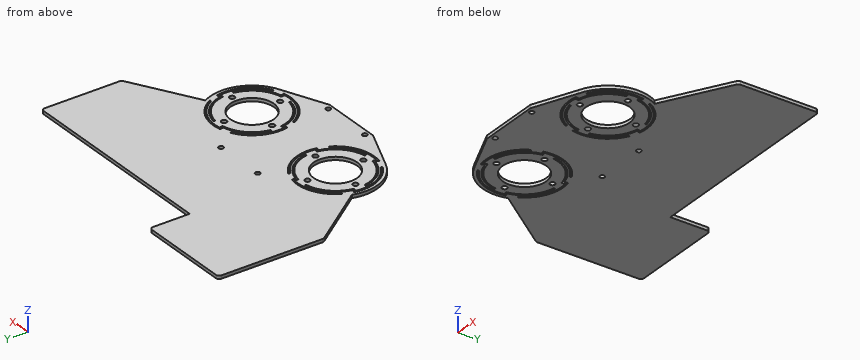
```python
from build123d import *

# Parameters (mm, degrees)
SKETCH_1_R          = 21
SKETCH_1_R_2        = 13.6
SKETCH_1_R_3        = 1.65
EXTRUDE_1_DEPTH     = 2
EXTRUDE_1_2_DEPTH   = 2
SKETCH_2_R          = 26.25
EXTRUDE_3_DEPTH     = 2
EXTRUDE_4_DEPTH     = 2
FILLET_1_R          = 2
SKETCH_4_R          = 1.5
CUT_EXTRUDE_1_DEPTH = 2


with BuildPart() as part:
    # Sketch 1 → Extrude 1 (new body)
    with BuildSketch(Plane.XY):
        with Locations((36.5, 0)):
            Circle(SKETCH_1_R)
        with Locations((36.5, 0)):
            Circle(SKETCH_1_R_2, mode=Mode.SUBTRACT)
        with Locations((19, 0)):
            Circle(SKETCH_1_R_3, mode=Mode.SUBTRACT)
        with Locations((36.5, 17.5)):
            Circle(SKETCH_1_R_3, mode=Mode.SUBTRACT)
        with Locations((54, 0)):
            Circle(SKETCH_1_R_3, mode=Mode.SUBTRACT)
        with Locations((36.5, -17.5)):
            Circle(SKETCH_1_R_3, mode=Mode.SUBTRACT)
    extrude(amount=EXTRUDE_1_DEPTH)

    # Sketch 2 → Extrude 3 (add)
    # profile 1 of 4: a face of its own
    with BuildSketch(Plane.XY):
        with Locations((36.5, 0)):
            Circle(SKETCH_2_R)
        with BuildLine():
            Line((58.229143493, 3.441558231), (57.241455152, 3.285123766))
            ThreePointArc((57.241455152, 3.285123766), (57.435264008, 1.64764101), (57.5, 0))
            ThreePointArc((57.5, 0), (57.435264008, -1.64764101), (57.241455152, -3.285123766))
            Line((57.241455152, -3.285123766), (58.229143493, -3.441558231))
            ThreePointArc((58.229143493, -3.441558231), (52.524161337, -15.074025787), (41.261671507, -21.478512157))
            Line((41.261671507, -21.478512157), (41.748660638, -23.675178173))
            ThreePointArc((41.748660638, -23.675178173), (26.251507153, -21.977963836), (14.989987295, -11.197403871))
            Line((14.989987295, -11.197403871), (15.876998129, -10.735655258))
            ThreePointArc((15.876998129, -10.735655258), (26.035211246, -20.761760434), (40.137101312, -22.963753919))
            Line((40.137101312, -22.963753919), (39.785123766, -20.741455152))
            ThreePointArc((39.785123766, -20.741455152), (36.5, -21), (33.214876234, -20.741455152))
            Line((33.214876234, -20.741455152), (33.058441769, -21.729143493))
            ThreePointArc((33.058441769, -21.729143493), (21.425974213, -16.024161337), (15.021487843, -4.761671507))
            Line((15.021487843, -4.761671507), (12.824821827, -5.248660638))
            ThreePointArc((12.824821827, -5.248660638), (14.522036164, 10.248492847), (25.302596129, 21.510012705))
            Line((25.302596129, 21.510012705), (25.764344742, 20.623001871))
            ThreePointArc((25.764344742, 20.623001871), (15.738239566, 10.464788754), (13.536246081, -3.637101312))
            Line((13.536246081, -3.637101312), (14.770856507, -3.441558231))
            Line((14.770856507, -3.441558231), (15.758544848, -3.285123766))
            ThreePointArc((15.758544848, -3.285123766), (15.5, 0), (15.758544848, 3.285123766))
            Line((15.758544848, 3.285123766), (14.770856507, 3.441558231))
            ThreePointArc((14.770856507, 3.441558231), (20.475838663, 15.074025787), (31.738328493, 21.478512157))
            Line((31.738328493, 21.478512157), (31.251339362, 23.675178173))
            ThreePointArc((31.251339362, 23.675178173), (46.748492847, 21.977963836), (58.010012705, 11.197403871))
            ThreePointArc((58.010012705, 11.197403871), (59.287546054, 8.293988476), (60.175178173, 5.248660638))
            ThreePointArc((60.175178173, 5.248660638), (58.477963836, -10.248492847), (47.697403871, -21.510012705))
            Line((47.697403871, -21.510012705), (47.235655258, -20.623001871))
            ThreePointArc((47.235655258, -20.623001871), (57.261760434, -10.464788754), (59.463753919, 3.637101312))
            Line((59.463753919, 3.637101312), (58.229143493, 3.441558231))
        make_face(mode=Mode.SUBTRACT)
    # profile 2 of 4: a face of its own
    with BuildSketch(Plane.XY):
        with BuildLine():
            Line((39.785123766, 20.741455152), (39.941558231, 21.729143493))
            ThreePointArc((39.941558231, 21.729143493), (51.574025787, 16.024161337), (57.978512157, 4.761671507))
            Line((57.978512157, 4.761671507), (60.175178173, 5.248660638))
            ThreePointArc((60.175178173, 5.248660638), (59.287546054, 8.293988476), (58.010012705, 11.197403871))
            Line((58.010012705, 11.197403871), (57.123001871, 10.735655258))
            ThreePointArc((57.123001871, 10.735655258), (46.964788754, 20.761760434), (32.862898688, 22.963753919))
            Line((32.862898688, 22.963753919), (33.214876234, 20.741455152))
            ThreePointArc((33.214876234, 20.741455152), (36.5, 21), (39.785123766, 20.741455152))
        make_face()
    # profile 3 of 4: a face of its own
    with BuildSketch(Plane.XY):
        with Locations((-36.5, 0)):
            Circle(SKETCH_2_R)
        with BuildLine():
            ThreePointArc((-31.738328493, 21.478512157), (-20.475838663, 15.074025787), (-14.770856507, 3.441558231))
            Line((-14.770856507, 3.441558231), (-15.758544848, 3.285123766))
            ThreePointArc((-15.758544848, 3.285123766), (-15.564735992, 1.64764101), (-15.5, 0))
            ThreePointArc((-15.5, 0), (-15.564735992, -1.64764101), (-15.758544848, -3.285123766))
            Line((-15.758544848, -3.285123766), (-14.770856507, -3.441558231))
            Line((-14.770856507, -3.441558231), (-13.536246081, -3.637101312))
            ThreePointArc((-13.536246081, -3.637101312), (-15.738239566, 10.464788754), (-25.764344742, 20.623001871))
            Line((-25.764344742, 20.623001871), (-25.302596129, 21.510012705))
            ThreePointArc((-25.302596129, 21.510012705), (-14.522036164, 10.248492847), (-12.824821827, -5.248660638))
            Line((-12.824821827, -5.248660638), (-15.021487843, -4.761671507))
            ThreePointArc((-15.021487843, -4.761671507), (-21.425974213, -16.024161337), (-33.058441769, -21.729143493))
            Line((-33.058441769, -21.729143493), (-33.214876234, -20.741455152))
            ThreePointArc((-33.214876234, -20.741455152), (-36.5, -21), (-39.785123766, -20.741455152))
            Line((-39.785123766, -20.741455152), (-40.137101312, -22.963753919))
            ThreePointArc((-40.137101312, -22.963753919), (-26.035211246, -20.761760434), (-15.876998129, -10.735655258))
            Line((-15.876998129, -10.735655258), (-14.989987295, -11.197403871))
            ThreePointArc((-14.989987295, -11.197403871), (-26.251507153, -21.977963836), (-41.748660638, -23.675178173))
            Line((-41.748660638, -23.675178173), (-41.261671507, -21.478512157))
            ThreePointArc((-41.261671507, -21.478512157), (-52.524161337, -15.074025787), (-58.229143493, -3.441558231))
            Line((-58.229143493, -3.441558231), (-57.241455152, -3.285123766))
            ThreePointArc((-57.241455152, -3.285123766), (-57.5, 0), (-57.241455152, 3.285123766))
            Line((-57.241455152, 3.285123766), (-58.229143493, 3.441558231))
            Line((-58.229143493, 3.441558231), (-59.463753919, 3.637101312))
            ThreePointArc((-59.463753919, 3.637101312), (-57.261760434, -10.464788754), (-47.235655258, -20.623001871))
            Line((-47.235655258, -20.623001871), (-47.697403871, -21.510012705))
            ThreePointArc((-47.697403871, -21.510012705), (-58.477963836, -10.248492847), (-60.175178173, 5.248660638))
            ThreePointArc((-60.175178173, 5.248660638), (-59.287546054, 8.293988476), (-58.010012705, 11.197403871))
            ThreePointArc((-58.010012705, 11.197403871), (-46.748492847, 21.977963836), (-31.251339362, 23.675178173))
            Line((-31.251339362, 23.675178173), (-31.738328493, 21.478512157))
        make_face(mode=Mode.SUBTRACT)
    # profile 4 of 4: a face of its own
    with BuildSketch(Plane.XY):
        with BuildLine():
            ThreePointArc((-39.785123766, 20.741455152), (-36.5, 21), (-33.214876234, 20.741455152))
            Line((-33.214876234, 20.741455152), (-32.862898688, 22.963753919))
            ThreePointArc((-32.862898688, 22.963753919), (-46.964788754, 20.761760434), (-57.123001871, 10.735655258))
            Line((-57.123001871, 10.735655258), (-58.010012705, 11.197403871))
            ThreePointArc((-58.010012705, 11.197403871), (-59.287546054, 8.293988476), (-60.175178173, 5.248660638))
            Line((-60.175178173, 5.248660638), (-57.978512157, 4.761671507))
            ThreePointArc((-57.978512157, 4.761671507), (-51.574025787, 16.024161337), (-39.941558231, 21.729143493))
            Line((-39.941558231, 21.729143493), (-39.785123766, 20.741455152))
        make_face()
    extrude(amount=EXTRUDE_3_DEPTH)


with BuildPart() as body_2:
    # Sketch 1 → Extrude 1 2 (new body)
    with BuildSketch(Plane.XY):
        with Locations(Location((-36.5, 0, 0), (0, 0, 180))):
            Circle(SKETCH_1_R)
        with Locations(Location((-36.5, -17.5, 0), (0, 0, 180))):
            Circle(SKETCH_1_R_3, mode=Mode.SUBTRACT)
        with Locations(Location((-54, 0, 0), (0, 0, 180))):
            Circle(SKETCH_1_R_3, mode=Mode.SUBTRACT)
        with Locations(Location((-36.5, 17.5, 0), (0, 0, 180))):
            Circle(SKETCH_1_R_3, mode=Mode.SUBTRACT)
        with Locations(Location((-19, 0, 0), (0, 0, 180))):
            Circle(SKETCH_1_R_3, mode=Mode.SUBTRACT)
        with Locations(Location((-36.5, 0, 0), (0, 0, 180))):
            Circle(SKETCH_1_R_2, mode=Mode.SUBTRACT)
    extrude(amount=EXTRUDE_1_2_DEPTH)


with BuildPart() as extrude_3_piece_1:
    # of the separate pieces the step leaves, piece 1, a body of its own (extrude_3_pieces)
    add(part.part.solids().sort_by_distance((57.241455152, 3.285123766, 0))[0])



with BuildPart() as extrude_3_piece_2:
    # of the separate pieces the step leaves, piece 2, a body of its own (extrude_3_pieces)
    add(part.part.solids().sort_by_distance((-10.25, 0, 0))[0])


with BuildPart() as extrude_3_piece_1_1:
    add(extrude_3_piece_1.part)

    add(extrude_3_piece_2.part)  # Extrude 4 merges Extrude 3 piece 2

    add(body_2.part)  # Extrude 4 merges body 2
    # Sketch 3 → Extrude 4 (add)
    with BuildSketch(Plane.XY):
        with BuildLine():
            Line((0, -36), (0, 0))
            Line((0, 0), (0, 86))
            Line((0, 86), (-29.25, 86))
            Line((-29.25, 86), (-29.25, 111))
            Line((-29.25, 111), (-89.25, 111))
            Line((-89.25, 111), (-89.25, 45))
            Line((-89.25, 45), (-61.597026322, 7.694268631))
            ThreePointArc((-61.597026322, 7.694268631), (-32.609912659, 25.960156403), (-10.25, 0))
            ThreePointArc((-10.25, 0), (-22.029919095, -21.90158119), (-46.796991132, -24.1461068))
            Line((-46.796991132, -24.1461068), (-19, -36))
            Line((-19, -36), (0, -36))
        make_face()
        with BuildLine():
            Line((0, 86), (0, 0))
            Line((0, 0), (0, -36))
            Line((0, -36), (19, -36))
            Line((19, -36), (45.243812785, -24.750923982))
            ThreePointArc((45.243812785, -24.750923982), (11.927256564, 9.232701664), (59.37885785, 12.86935754))
            Line((59.37885785, 12.86935754), (100.5, 36))
            Line((100.5, 36), (100.5, 86))
            Line((100.5, 86), (29.25, 86))
            Line((29.25, 86), (0, 86))
        make_face()
    extrude(amount=EXTRUDE_4_DEPTH)

    # Fillet 1
    fillet_1_edges = [extrude_3_piece_1_1.edges().sort_by_distance(p)[0] for p in [
        (-19, -36, 1),
        (19, -36, 1),
        (100.5, 36, 1),
        (100.5, 86, 1),
        (-29.25, 111, 1),
        (-89.25, 111, 1),
        (-89.25, 45, 1),
    ]]
    fillet(fillet_1_edges, radius=FILLET_1_R)

    # Sketch 4 → Cut-Extrude 1 (cut)
    with BuildSketch(Plane.XY.offset(2)):
        with Locations((-16, -33)):
            Circle(SKETCH_4_R)
        with Locations((16, -33)):
            Circle(SKETCH_4_R)
        with Locations((-16, 34)):
            Circle(SKETCH_4_R)
        with Locations((16, 34)):
            Circle(SKETCH_4_R)
    extrude(amount=-CUT_EXTRUDE_1_DEPTH, mode=Mode.SUBTRACT)


solid = extrude_3_piece_1_1.part
```
Can you work these out from the model? Positions are in its coordinate system, mm. Coordinates: 2 decimals unless noted, no trailing zeros. Write each loop counter-clockwise with the first axis right and the second up, starting at its lowest first coordinate (ties: lowest second). Pieces come first, ordered by that corner, then holes. Notation, with made-up numbers: M -40,68 L -29,68 A15 ccw -29,91 Z; hole C 69.25,46 d6. An arc over 180 degrees is marked long. Answer as CSV lines item,"result".
Item 1: Imagine slicing it at A-A on z = 0.45. State how many separate pieces and enclosed holes the cut face has, plus the area to 3 significant figures.
Geometry results:
separate pieces,"1"
enclosed holes,"22"
area,"18,000 mm2"
Item 2: Imagine slicing it at B-B on x = 0. List the corners of the cut face in (y, z) for me.
Geometry results:
outline,"M -36,0 L 86,0 L 86,2 L -36,2 Z"
Item 3: I'm going to push flat-ended pins straight in: P1, Ø6, axis at x = 73, y = 22, coming from the -Z side; P2, Ø1, axis at y = 100, z = 0.5, coming from the +X side. Where does each tip first touch, or does it pass through?
Geometry results:
P1,"stops at z = 0"
P2,"stops at x = -29.25"
Item 4: Imagine slicing it at C-C on y = 97.5. List the corners of the cut face in (x, z) for me.
Geometry results:
outline,"M -89.25,0 L -29.25,0 L -29.25,2 L -89.25,2 Z"
Item 5: Please list where these lines run through material, in increasing order: line 1 along Y through (x, z) = (45, 0.65); line 2 along Y through (x, z) = (-36.5, 1.55); line 3 along Y through (x, z) = (-52, 1.3).
Geometry results:
line 1,"y = -24.86 to -20.29, -19.2 to -10.62, 10.62 to 19.2, 20.29 to 21.64, 22.71 to 86"
line 2,"y = -28.54 to -24.25, -23.25 to -19.15, -15.85 to -13.6, 13.6 to 15.85, 19.15 to 23.25, 24.25 to 111"
line 3,"y = -21.19 to -18.65, -17.33 to -15.61, -14.17 to 14.17, 15.61 to 17.33, 18.65 to 111"
